Geometry check sheet. Reference: the model listing, model coordinates, mm. A direction names the side the tool comes from. Coordinates: 2 decimals unless noted, no trailing zeros. Write each loop counter-clockwise with the first axis right and the second up, starting at its lowest first coordinate (ties: lowest second). Pieces come first, ordered by that corner, then holes. Notation, with made-up numbers: (63, 68.25) -> (70, 68.25) arc R13 cw to (70, 89.25) -> close; hole circle Ø6 at (-16, 0). An arc over 180 degrees is marked (long way). Answer in a Markdown table with one row per item. Add a question column.
Q1. Section check C-C, the plane y = 2.45. Record the boundary of the cut face in (x, z), and give its area (3 significant figures).
Q2. Thickness scan on line 1 (Y direction, x = 1.75, z = 0.5); line 2 (X direction, y = 2.6, z = 9); line 3 (X direction, y = 0.9, z = 0.75). Record the ranges inside material, lowest first.
Q3. Tool access check on faces 1 (the face through (4.5, 3, 4.9)), 2 (the face through (4, 2.5, 4.9)). Record the directions out of +Z, -Z, +X, -X, +Y, -Y that give a thin tool (end or side, any length) a straight path to the whole face; none if there is none.
Q4. Section check B-B, the plane x = -11.75. Record the boundary of the cut face in (y, z).
Q5. Section check A-A, the plane z = 3.75. Record the boundary of the cut face in (x, y), and give its area (3 significant figures).
Q6. Gauge pin test, flat end, axial feed: P1, Ø1, axis at x = -21.5, z = 6.5, coming from the +Y side. Record the tip position at first contact, or that the pin passes through.
```python
from build123d import *

# Parameters (mm, degrees)
BOSS_EXTRUDE1_DEPTH = 10
FILLET1_R           = 2
SKETCH3_R           = 0.25
CUT_EXTRUDE1_DEPTH  = 11


with BuildPart() as part:
    # Sketch1 → Boss-Extrude1 (new body)
    with BuildSketch(Plane.XY):
        Polygon((4, 3), (5, 3), (5, -1), (-25, -1), (-25, 0), (4, 0), align=None)
    extrude(amount=BOSS_EXTRUDE1_DEPTH)

    # Fillet1
    fillet1_edges = [part.edges().sort_by_distance(p)[0] for p in [
        (4, 0, 5),
    ]]
    fillet(fillet1_edges, radius=FILLET1_R)

    # Sketch3 → Cut-Extrude1 (cut, through all)
    with BuildSketch(Plane.XY.offset(10)):
        with Locations((-24.436460419, -0.529384592)):
            Circle(SKETCH3_R)
    extrude(amount=-CUT_EXTRUDE1_DEPTH, mode=Mode.SUBTRACT)


solid = part.part
```
Calculated:
| question | item | result |
|---|---|---|
| 1 | outline | (4, 0) -> (5, 0) -> (5, 10) -> (4, 10) -> close |
| 1 | area | 10.0 mm² |
| 2 | line 1 | y = -1 to 0 |
| 2 | line 2 | x = 4 to 5 |
| 2 | line 3 | x = 3.67 to 5 |
| 3 | face 1 | +Z, -Z, +X, -X, +Y |
| 3 | face 2 | +Z, -Z, -X, +Y |
| 4 | outline | (-1, 0) -> (0, 0) -> (0, 10) -> (-1, 10) -> close |
| 5 | outline | (-25, -1) -> (5, -1) -> (5, 3) -> (4, 3) -> (4, 2) arc R2 cw to (2, 0) -> (-25, 0) -> close; hole circle Ø0.5 at (-24.44, -0.53) |
| 5 | area | 33.7 mm² |
| 6 | P1 | stops at y = 0 |
